Geometry check sheet. Reference: the model listing, model coordinates, mm. A direction names the side the tool comes from. Give positions to 0.01 mm unless a question says otherwise; leave off trailing zeros. Loops run counter-clockwise (first coordinate to the right, second up) from the corner with the lowest first, then second, coordinate; pieces in that order, holes last.
1. Cross-section at A-A, the plane z = 36.5. Record the cut outline in (x, y), plus the area to 3 significant figures.
2. Material ranges on L1, parallel to Y at x = -54, z = 32; L2, parallel to Z at x = 30.5, y = -17; L3, parallel to Y at x = 62, z = 45.5, recorded low to high.
3. Cross-section at D-D, the plane x = -43. Record the cut outline in (y, z), plus the area to 3 significant figures.
4. Go/stop test with flat-tipped pins: pin 1 Ø23 at (x, y) = (11.5, -50.5) entering from -Z; pin 2 Ø12 at (x, y) = (-41.5, -32) entering from +Z. Record where each tip stops, or that it passes through.
5. Cross-section at B-B, the plane y = -18.5. Record the cut outline in (x, z), plus the area to 3 significant figures.
6. Tool access check on faces 1 (the flat face through (1, -25.4, 44)), 2 (the flat face through (45.89, -38.63, 6.26)), 3 (the flat face through (1, -57, 38.1)). Record the directions out of +Z, -Z, +X, -X, +Y, -Y that give a thin tool (end or side, any length) a straight path to the whole face; none if there is none.
7. Cross-section at C-C, the plane x = 12.5. Record the cut outline in (y, z), plus the area to 3 significant figures.
8. Release check for a two-part mould opening along Y. For faces 4 (the flat face through (1, -63.5, 32)), 5 (the flat face through (-1, 0, 26)), 6 (the flat face through (-1, -63, 50.8)), 7 (the flat face through (-1, -76.2, 26)) record: +Y half, -Y half, draft (parallel to the pull), parting line (faces both ways), or undercut.
from build123d import *

# Parameters (mm, degrees)
F0_W     = 152.4
F0_H     = 50.8
F1_DEPTH = 76.2
F3_DEPTH = 76.2
F5_DEPTH = 152.4


with BuildPart() as f1:
    # F0 (on Front) → F1 (new body)
    with BuildSketch(Plane.XZ):
        with Locations((-0.068524, 25.4)):
            Rectangle(F0_W, F0_H)
    extrude(amount=F1_DEPTH)

    # F2 (on face) → F3 (cut, through all)
    with BuildSketch(Plane.XZ.offset(76.2)):
        Polygon((0, 12.7), (0, 0), (41.121963, 0), (50.8, 12.7), align=None)
        Polygon((-41.190486, 0), (0, 0), (0, 12.7), (-50.8, 12.7), align=None)
    extrude(amount=-F3_DEPTH, mode=Mode.SUBTRACT)

    # F4 (on face) → F5 (cut, through all)
    with BuildSketch(Plane.YZ.offset(76.131476)):
        Polygon((-63.5, 25.4), (-12.7, 25.4), (-12.7, 38.1), (-25.4, 38.1), (-25.4, 50.8), (-49.570005, 50.8), (-50.8, 50.8), (-50.8, 38.1), (-63.5, 38.1), align=None)
    extrude(amount=-F5_DEPTH, mode=Mode.SUBTRACT)


solid = f1.part
Result:
1. outline: (-76.27, -76.2) - (76.13, -76.2) - (76.13, -63.5) - (-76.27, -63.5) - close; (-76.27, -12.7) - (76.13, -12.7) - (76.13, 0) - (-76.27, 0) - close
1. area: 3,870 mm2
2. L1: y = -76.2 to -63.5, -12.7 to 0
2. L2: z = 12.7 to 25.4, 38.1 to 50.8
2. L3: y = -76.2 to -50.8, -25.4 to 0
3. outline: (-76.2, 0) - (0, 0) - (0, 2.39) - (-76.2, 2.39) - close; (-76.2, 12.7) - (0, 12.7) - (0, 50.8) - (-25.4, 50.8) - (-25.4, 38.1) - (-12.7, 38.1) - (-12.7, 25.4) - (-63.5, 25.4) - (-63.5, 38.1) - (-50.8, 38.1) - (-50.8, 50.8) - (-76.2, 50.8) - close
3. area: 2,120 mm2
4. pin 1: stops at z = 12.7
4. pin 2: stops at z = 25.4
5. outline: (-76.27, 0) - (-41.19, 0) - (-50.8, 12.7) - (50.8, 12.7) - (41.12, 0) - (76.13, 0) - (76.13, 25.4) - (-76.27, 25.4) - close; (-76.27, 38.1) - (76.13, 38.1) - (76.13, 50.8) - (-76.27, 50.8) - close
5. area: 4,640 mm2
6. face 1: +Z, +X, -X
6. face 2: +Y, -Y
6. face 3: +X, -X
7. outline: (-76.2, 12.7) - (0, 12.7) - (0, 50.8) - (-25.4, 50.8) - (-25.4, 38.1) - (-12.7, 38.1) - (-12.7, 25.4) - (-63.5, 25.4) - (-63.5, 38.1) - (-50.8, 38.1) - (-50.8, 50.8) - (-76.2, 50.8) - close
7. area: 1,940 mm2
8. face 4: undercut
8. face 5: +Y half
8. face 6: draft
8. face 7: -Y half
